Here's how the part is built. I have some questions about the finished solid (model axes, mm). A direction names the side the tool comes from. Give positions to 0.01 mm unless a question says otherwise; leave off trailing zeros. Loops run counter-clockwise (first coordinate to the right, second up) from the corner with the lowest first, then second, coordinate; pieces in that order, holes last.
Q1. I'm going to push flat-ended pins straight in: P1, Ø2, axis at y = 25, z = 7, coming from the +X side; P2, Ø1.3, axis at y = 31.5, z = 4, coming from the +X side. Where does each tip first touch, or does it pass through?
Q2. I need wall thicknesses on probe 1 along Y at (x, z) = (-161.5, 6.25); probe 2 along Z at (x, y) = (-186.5, 14.5); probe 3 along X at (y, z) = (25.5, 4.5). Which ranges of each line are inside material? Lowest first, please.
Q3. Suppose I cut it at D-D (x = -163). List the corners of the cut face in (y, z) for me.
Q4. Suppose I cut it at B-B (z = 2.75). List the corners of the cut face in (x, y) for me.
Q5. Thinking about a two-plate mould opening in Z: for faces 4 (the face through (-157.424, 10, 7)), 5 (the face through (-157.72, 39.35, 8.21)), 6 (the face through (-186, 24, 6.5)), which applies, pulls with the +Z half, pulls with the -Z half, needs draft (parallel to the pull), parting line crosses it, or undercut?
Q6. Suppose I cut it at A-A (x = -186). List the corners of the cut face in (y, z) for me.
Q7. For faces 1 (the face through (-172, 38.332, 7)), 2 (the face through (-173.23, 7.63, 8.21)), 3 (the face through (-172, 9.332, 4)), which set-ups out of +Z, -Z, +X, -X, +Y, -Y let a thin tool reach every point of the face, with its end or its side?
Q8. Suppose I cut it at C-C (y = 32.5). List the corners of the cut face in (x, z) for me.
```python
from build123d import *

# Parameters (mm, degrees)
SKETCH1_W           = 32
SKETCH1_H           = 35
BOSS_EXTRUDE1_DEPTH = 2
BOSS_EXTRUDE2_DEPTH = 4.5
BOSS_EXTRUDE3_DEPTH = 2
FILLET1_START       = -1
FILLET1_DEPTH       = 10
FILLET2_R           = 1


with BuildPart() as part:
    # Sketch1 → Boss-Extrude1 (new body)
    with BuildSketch(Plane.XY):
        with Locations((-173.423957437, 24.831611866)):
            Rectangle(SKETCH1_W, SKETCH1_H)
    extrude(amount=BOSS_EXTRUDE1_DEPTH)

    # Sketch2 → Boss-Extrude2 (add)
    with BuildSketch(Plane.XY.offset(2)):
        Polygon((-157.423957437, 42.331611866), (-189.423957437, 42.331611866), (-189.423957437, 7.331611866), (-157.423957437, 7.331611866), (-157.423957437, 9.331611866), (-187.423957437, 9.331611866), (-187.423957437, 40.331611866), (-157.423957437, 40.331611866), align=None)
    extrude(amount=BOSS_EXTRUDE2_DEPTH)

    # Sketch3 → Boss-Extrude3 (add)
    with BuildSketch(Plane.XY.offset(6.5)):
        Polygon((-157.423957437, 42.331611866), (-189.423957437, 42.331611866), (-189.423957437, 7.331611866), (-157.423957437, 7.331611866), (-157.423957437, 11.331611866), (-185.423957437, 11.331611866), (-185.423957437, 38.331611866), (-157.423957437, 38.331611866), align=None)
    extrude(amount=BOSS_EXTRUDE3_DEPTH)

    # Fillet1: read off the stored shape, not the designer's step
    # Fillet1 outline → Fillet1 (cut)
    with BuildSketch(Plane.XY.offset(FILLET1_START)):
        with BuildLine():
            Line((-157.423957437, 42.331611866), (-159.423957437, 42.331611866))
            ThreePointArc((-159.423957437, 42.331611866), (-158.009743875, 41.745825428), (-157.423957437, 40.331611866))
            Line((-157.423957437, 40.331611866), (-157.423957437, 42.331611866))
        make_face()
        with BuildLine():
            ThreePointArc((-189.423957437, 40.331611866), (-188.838170999, 41.745825428), (-187.423957437, 42.331611866))
            Line((-187.423957437, 42.331611866), (-189.423957437, 42.331611866))
            Line((-189.423957437, 42.331611866), (-189.423957437, 40.331611866))
        make_face()
        with BuildLine():
            ThreePointArc((-187.423957437, 7.331611866), (-188.838170999, 7.917398304), (-189.423957437, 9.331611866))
            Line((-189.423957437, 9.331611866), (-189.423957437, 7.331611866))
            Line((-189.423957437, 7.331611866), (-187.423957437, 7.331611866))
        make_face()
        with BuildLine():
            Line((-157.423957437, 7.331611866), (-157.423957437, 9.331611866))
            ThreePointArc((-157.423957437, 9.331611866), (-158.009743875, 7.917398303), (-159.423957437, 7.331611866))
            Line((-159.423957437, 7.331611866), (-157.423957437, 7.331611866))
        make_face()
    extrude(amount=FILLET1_DEPTH, mode=Mode.SUBTRACT)

    # Fillet2
    fillet2_edges = [part.edges().sort_by_distance(p)[0] for p in [
        (-157.423957437, 10.331611866, 8.5),
        (-158.009743875, 41.745825428, 8.5),
        (-173.423957437, 42.331611866, 8.5),
        (-188.838170999, 41.745825428, 8.5),
        (-158.009743875, 7.917398303, 8.5),
        (-173.423957437, 7.331611866, 8.5),
        (-188.838170999, 7.917398304, 8.5),
        (-189.423957437, 24.831611866, 8.5),
    ]]
    fillet(fillet2_edges, radius=FILLET2_R)


solid = part.part
```
Solutions:
1. P1: stops at x = -185.42
1. P2: stops at x = -187.42
2. probe 1: y = 7.33 to 9.33, 40.33 to 42.33
2. probe 2: z = 0 to 2, 6.5 to 8.5
2. probe 3: x = -189.42 to -187.42
3. outline: (7.33, 0) - (42.33, 0) - (42.33, 7.5) arc R1 ccw to (41.33, 8.5) - (38.33, 8.5) - (38.33, 6.5) - (40.33, 6.5) - (40.33, 2) - (9.33, 2) - (9.33, 6.5) - (11.33, 6.5) - (11.33, 8.5) - (8.33, 8.5) arc R1 ccw to (7.33, 7.5) - close
4. outline: (-189.42, 9.33) arc R2 ccw to (-187.42, 7.33) - (-159.42, 7.33) arc R2 ccw to (-157.42, 9.33) - (-187.42, 9.33) - (-187.42, 40.33) - (-157.42, 40.33) arc R2 ccw to (-159.42, 42.33) - (-187.42, 42.33) arc R2 ccw to (-189.42, 40.33) - close
5. face 4: needs draft
5. face 5: pulls with the +Z half
5. face 6: undercut
6. outline: (7.33, 0) - (42.33, 0) - (42.33, 7.5) arc R1 ccw to (41.33, 8.5) - (8.33, 8.5) arc R1 ccw to (7.33, 7.5) - close; hole (9.33, 2) - (40.33, 2) - (40.33, 6.5) - (9.33, 6.5) - close
7. face 1: +Z, +X
7. face 2: +Z, +X, -X, -Y
7. face 3: +X
8. outline: (-189.42, 0) - (-157.42, 0) - (-157.42, 2) - (-187.42, 2) - (-187.42, 6.5) - (-185.42, 6.5) - (-185.42, 8.5) - (-188.42, 8.5) arc R1 ccw to (-189.42, 7.5) - close
